```python
from build123d import *

# Parameters (mm, degrees)
SKETCH1_R           = 5
BOSS_EXTRUDE1_DEPTH = 1
SKETCH3_W           = 6
SKETCH3_H           = 16.269445872
CUT_EXTRUDE1_DEPTH  = 10


with BuildPart() as part:
    # Sketch1 → Boss-Extrude1 (new body)
    with BuildSketch(Plane.XY):
        Polygon((0, 45), (0, 36.742346142), (11.64685703, 43.466662183), (9.509618943, 35.490381057), (22.5, 38.97114317), (18.371173071, 31.819805153), (31.819805153, 31.819805153), (25.980762114, 25.980762114), (38.97114317, 22.5), (31.819805153, 18.371173071), (43.466662183, 11.64685703), (35.490381057, 9.509618943), (45, 0), (36.742346142, 0), (43.466662183, -11.64685703), (35.490381057, -9.509618943), (38.97114317, -22.5), (31.819805153, -18.371173071), (31.819805153, -31.819805153), (25.980762114, -25.980762114), (22.5, -38.97114317), (18.371173071, -31.819805153), (11.64685703, -43.466662183), (9.509618943, -35.490381057), (0, -45), (0, -36.742346142), (-11.64685703, -43.466662183), (-9.509618943, -35.490381057), (-22.5, -38.97114317), (-18.371173071, -31.819805153), (-31.819805153, -31.819805153), (-25.980762114, -25.980762114), (-38.97114317, -22.5), (-31.819805153, -18.371173071), (-43.466662183, -11.64685703), (-35.490381057, -9.509618943), (-45, 0), (-36.742346142, 0), (-43.466662183, 11.64685703), (-35.490381057, 9.509618943), (-38.97114317, 22.5), (-31.819805153, 18.371173071), (-31.819805153, 31.819805153), (-25.980762114, 25.980762114), (-22.5, 38.97114317), (-18.371173071, 31.819805153), (-11.64685703, 43.466662183), (-9.509618943, 35.490381057), align=None)
        Circle(SKETCH1_R, mode=Mode.SUBTRACT)
    extrude(amount=BOSS_EXTRUDE1_DEPTH)

    # Sketch3 → Cut-Extrude1 (cut)
    with BuildSketch(Plane.XY.offset(1)):
        with Locations((0, 0.439123073)):
            Rectangle(SKETCH3_W, SKETCH3_H)
    extrude(amount=-CUT_EXTRUDE1_DEPTH, mode=Mode.SUBTRACT)


solid = part.part
```
Design review of the part built by this model. Coordinates are the model's own, in mm. A direction names the side the tool comes from. Give positions to 0.01 mm unless a question says otherwise; leave off trailing zeros. Order: outer loops, then holes, each group sorted by start corner. A loop starts at its lowest first (then second) coordinate and runs counter-clockwise, first axis right, second up. Notation, with made-up numbers: (1.5, 26) -> (42.5, 26) arc R11 ccw to (42.5, 35) -> close; hole circle Ø6 at (65.5, 11.5). An arc over 180 degrees is marked (long way). Write item = value, one per line. Start each with the question number.
(1) We need section D-D on x = 15. Write out the cut boundary in (y, z), plus the area to 3 significant figures.
(2) We need section C-C on y = 13. Write out the cut boundary in (x, z).
(3) We need section B-B on x = 33. Write out the cut boundary in (y, z).
(4) For faces 4 (the face through (-15.056, 37.562, 0.493)), 5 (the face through (-10.59, -39.53, 0.49)), 6 (the face through (-39.53, -10.59, 0.49)), list the 3-axis set-ups (+Z, -Z, +X, -X, +Y, -Y) from which the entire face can be reached by the end or side of a thin tool; tool diameter is ignored.
(5) Mouldability with a two-part tool opening along Y and no side actions: class faces 1 (the face through (-28.9, 28.9, 0.5)), 2 (the face through (39.53, -10.59, 0.49)), 3 (the face through (-5.742, -40.057, 0.493)) as +Y half, -Y half, draft (parallel to the pull), parting line (faces both ways), or undercut.
(6) To check wall thickness, follow line 1 along X through (y, z) = (-41, 0.5); line 2 along X through (y, z) = (-30, 0.35); line 3 along Y through (x, z) = (34, 0.25). State the ranges of each line that lie inside material, in increasing order.
(7) We need section A-A on y = 29. Write out the cut boundary in (x, z), plus the area to 3 significant figures.
(8) For pin 1 (0.5 mm diameter, centred on y = -6.5, z = 0.5, fed in from +X); pin 2 (0.5 mm diameter, centred on y = -40, z = 0.5, fed in from -X); pin 3 (0.5 mm diameter, centred on x = -28.5, z = 0.5, fed in from -Y), all flat-tipped, find the tip position at first contact; note any pin that passes through.
Numbers:
q1.outline = (-37.66, 0) -> (36.96, 0) -> (36.96, 1) -> (-37.66, 1) -> close
q1.area = 74.6 mm^2
q2.outline = (-36.43, 0) -> (41.12, 0) -> (41.12, 1) -> (-36.43, 1) -> close
q3.outline = (-19.05, 0) -> (17.69, 0) -> (17.69, 1) -> (-19.05, 1) -> close; (19.05, 0) -> (24.1, 0) -> (24.1, 1) -> (19.05, 1) -> close
q4.face_4 = +Z, -Z, +Y
q4.face_5 = +Z, -Z
q4.face_6 = +Z, -Z, -X
q5.face_1 = +Y half
q5.face_2 = undercut
q5.face_3 = -Y half
q6.line_1 = -10.99 to -7.37, 0 to 4, 10.99 to 13.07
q6.line_2 = -30 to 24.9, 30 to 31.82
q6.line_3 = -19.63 to 17.11, 19.63 to 23.83
q7.outline = (-31.82, 0) -> (-29, 0) -> (-29, 1) -> (-31.82, 1) -> close; (-25.17, 0) -> (29, 0) -> (29, 1) -> (-25.17, 1) -> close
q7.area = 57.0 mm^2
q8.pin_1 = 40.64
q8.pin_2 = -10.78
q8.pin_3 = -31.82
